Answer from the drawing. Dimensions are ordinates in mm from the lowest x, y and z of the part. A direction names the side the tool comes from. Round coordinates to 2 decimals unless told otherwise and drop trailing zeros. Write each loop counter-clockwise with the first axis right and the second up, starting at its lowest first coordinate (ties: lowest second). Pieces come first, ordered by that corner, then holes. Notation, with made-up numbers: (57, 44) -> (100, 44) arc R10 cw to (100, 51) -> close; hole circle Ø8 at (7.25, -36.5). An arc over 180 degrees is marked (long way). Return JSON: item names as keys, results as strings. Group by question number.
(1) A cutting plane is placed at A-A on x = 2.54. Give the vertices of the cut face in (y, z) (1 decimal).
(2) Given pin 1 (3 mm diameter, centred on x = 37.5, z = 15, fed in from +Y) (1 decimal); pin 2 (4.5 mm diameter, centred on x = 50.5, z = 9, fed in from +Y); pin 3 (1.5 mm diameter, centred on y = 17.5, z = 9, fed in from -X); pin 4 (4 mm diameter, centred on x = 51.562, z = 5.08, fed in from +Y), each flat-ended and moving along its own axis, determine where each tip first touches the part or whether it passes through.
(3) A cutting plane is placed at D-D on y = 42. Give the vertices of the cut face in (x, z) (1 decimal).
(4) A cutting plane is placed at B-B on x = 25. Give the vertices of the cut face in (y, z) (1 decimal).
(5) For the marked faces 1, 2, 3 and 4, determine the directions among +Z, -Z, +X, -X, +Y, -Y from which every point of the face is accessible in a straight line to the end or side of a thin tool.
(6) Straight lines are drawn through the part: line 1 (Z direction, x = 2.54, y = 29.65) (1 decimal); line 2 (X direction, y = 29.5, z = 4); line 3 (Y direction, x = 29.5, z = 16.25). For each, find the intervals that lie inside material, in ascending order.
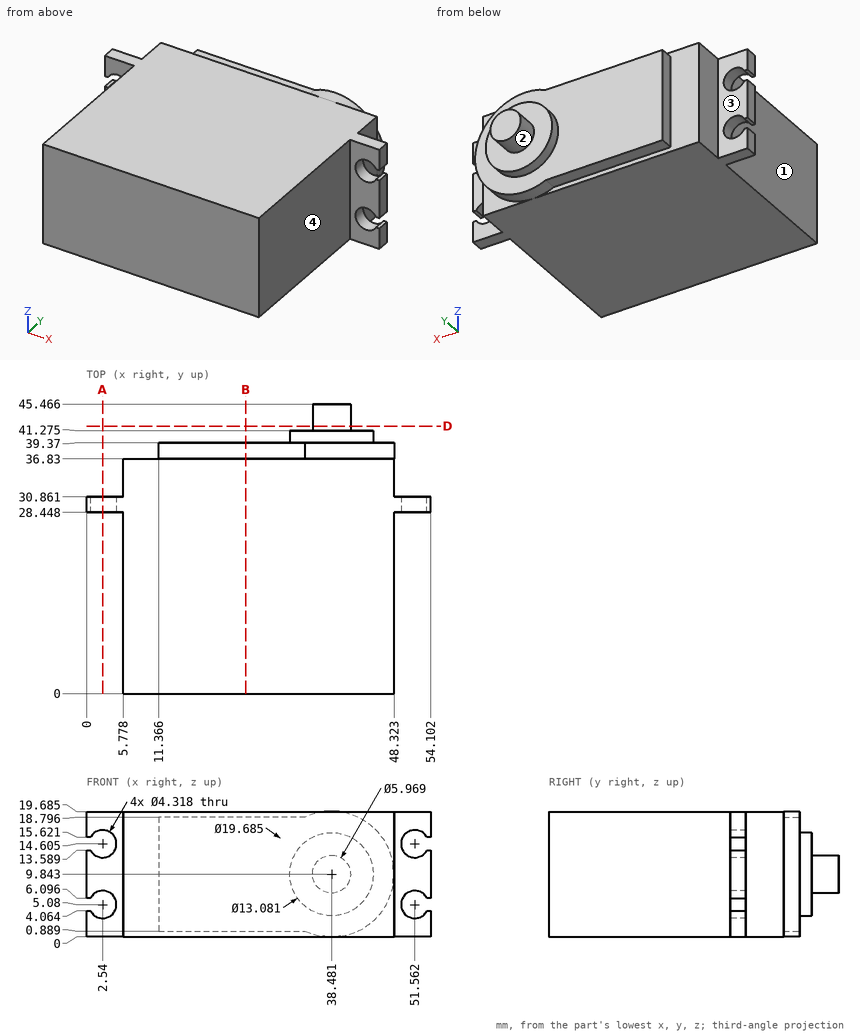
Checks:
{
 "1": {"outline": "(28.4, 0) -> (30.9, 0) -> (30.9, 2.9) -> (28.4, 2.9) -> close; (28.4, 7.2) -> (30.9, 7.2) -> (30.9, 12.4) -> (28.4, 12.4) -> close; (28.4, 16.8) -> (30.9, 16.8) -> (30.9, 19.7) -> (28.4, 19.7) -> close"},
 "2": {"pin 1": "stops at y = 41.3", "pin 2": "stops at y = 39.37", "pin 3": "stops at x = 5.78", "pin 4": "passes through"},
 "3": {"outline": "circle Ø6 at (38.5, 9.8)"},
 "4": {"outline": "(0, 0) -> (36.8, 0) -> (36.8, 0.9) -> (39.4, 0.9) -> (39.4, 18.8) -> (36.8, 18.8) -> (36.8, 19.7) -> (0, 19.7) -> close"},
 "5": {"face 1": "+Z, -Z, -X, -Y", "face 2": "+Y", "face 3": "+Z, -Z, -X, +Y", "face 4": "+Z, -Z, +X, -Y"},
 "6": {"line 1": "z = 0 to 2.9, 7.2 to 12.4, 16.8 to 19.7", "line 2": "x = 0 to 0.67, 4.41 to 49.69, 53.43 to 54.1", "line 3": "y = 0 to 39.37"}
}
